Geometry: final body of the model. Coordinates: model frame, mm. Face numbers are marked on the shaded views. A direction names the side the tool comes from. Coordinates: 2 decimals unless noted, no trailing zeros. Loops run counter-clockwise (first coordinate to the right, second up) from the corner with the lowest first, then second, coordinate; pieces in that order, holes last. Notation, with made-up numbers: (-23.75, -11) -> (7.25, -11) arc R20 ccw to (7.25, 23) -> close; hole circle Ø10 at (70, 42.25). An arc over 180 degrees is marked (long way). One line per item, written item: value. Start each with the question number.
Item 1: Contact query for flat-ended pins moving along their axis: pin 1 Ø3 at (x, y) = (29, -34) entering from +Z; pin 2 Ø3 at (x, z) = (-4, 28) entering from -Y; pin 3 Ø2 at (x, y) = (47.5, -15) entering from -Z; pin 4 Ø15 at (x, z) = (0, 0) entering from -Y. Output: stop coordinate, or through.
Item 2: Section query D-D on z = -17. Return loops of the section in (x, y).
Item 3: Section query A-A on x = 0. Return loops of the section in (y, z), then the cut area to 3 significant figures.
Item 4: Mould query, pull axis Y, two halves, no side actions, for the marked faces 5, 6, 7 and 8. Classes: +Y half, -Y half, draft (parallel to the pull), parting line (faces both ways), or undercut.
Item 5: Section query C-C on y = -25.4. Give the number of separate pieces and of enclosed holes in the cut face, then the cut area to 3 significant figures.
Item 6: Set-up query: the marked faces 1, 2, 3 and 4. Return all of +Z, -Z, +X, -X, +Y, -Y with unobstructed straight access to the full face (end or side cutting, diameter ignored); none if empty.
Item 7: Ray query, probe 1 along Y at (x, z) = (0, 96); probe 2 along Z at (x, y) = (88, -27); probe 3 along X at (y, z) = (-25, 76). Return the intervals inside material, ascending. Write a range as from..to.
Item 8: Section query B-B on z = 68. Return loops of the section in (x, y).
from build123d import *

# Parameters (mm, degrees)
F1_DEPTH  = 50.8
F2_R      = 63.5
F3_DEPTH  = 49.53
F4_R      = 8.3185
F5_DEPTH  = 25.4
F9_R      = 19.05
F11_DEPTH = 76.2
F10_R     = 19.05
F12_DEPTH = 76.2
F6_R      = 19.05
F13_DEPTH = 76.2
F7_R      = 19.05
F14_DEPTH = 76.2
F8_R      = 19.05
F15_DEPTH = 76.2
F16_R     = 19.05


# Not quite as in the source:
# - a feature names something its author has since deleted; it is built from what else it names


with BuildPart() as f1:
    # F0 (on Front) → F1 (new body)
    with BuildSketch(Plane.XZ):
        Polygon((-23.0722505283, 63.5), (-46.1354505283, 63.5), (-53.262371273, 41.5655933534), (-113.6544600578, 61.1881724962), (-127.9083015471, 17.319359203), (-67.5218062965, -2.3204350678), (-74.6487270411, -24.2548417144), (-55.9902062965, -37.8110505451), (-93.314569817, -89.1836296879), (-55.9828842652, -116.3066868834), (-18.6585207447, -64.9341077406), (0, -78.4903165712), (18.6585207447, -64.9341077406), (55.9828842652, -116.3066868834), (93.2999257546, -89.194269222), (55.9902062965, -37.8110505451), (74.6487270411, -24.2548417144), (67.5218062965, -2.3204350678), (127.9138950812, 17.302144075), (113.6564223157, 61.1821332873), (53.2643335309, 41.5595541445), (46.1354505283, 63.5), (23.0722505283, 63.5), (23.0722505283, 127), (-23.0722505283, 127), align=None)
    extrude(amount=F1_DEPTH)

    # F2 (on face) → F3 (cut)
    with BuildSketch(Plane.XZ.offset(50.8)):
        Circle(F2_R)
    extrude(amount=-F3_DEPTH, mode=Mode.SUBTRACT)

    # F4 (on face) → F5 (cut)
    with BuildSketch(Plane(origin=(0, 0, 0), x_dir=(-1, 0, 0), z_dir=(0, 1, 0))):
        Circle(F4_R)
    extrude(amount=-F5_DEPTH, mode=Mode.SUBTRACT)

    # F9 (on face) → F11 (cut)
    with BuildSketch(Plane(origin=(-74.6487270411, 0, -102.7451582856), x_dir=(0.8090169944, 0, -0.5877852523), z_dir=(-0.5877852523, 0, -0.8090169944))):
        with Locations((0, 25.4)):
            Circle(F9_R)
    extrude(amount=-F11_DEPTH, mode=Mode.SUBTRACT)

    # F10 (on face) → F12 (cut)
    with BuildSketch(Plane(origin=(-120.7841775695, 0, 39.2451582856), x_dir=(0, -1, 0), z_dir=(-0.9510565163, 0, 0.3090169944))):
        with Locations((25.4, 0)):
            Circle(F10_R)
    extrude(amount=-F12_DEPTH, mode=Mode.SUBTRACT)

    # F6 (on face) → F13 (cut)
    with BuildSketch(Plane.XY.offset(127)):
        with Locations((0, -25.4)):
            Circle(F6_R)
    extrude(amount=-F13_DEPTH, mode=Mode.SUBTRACT)

    # F7 (on face) → F14 (cut)
    with BuildSketch(Plane(origin=(120.7841775695, 0, 39.2451582856), x_dir=(0, 1, 0), z_dir=(0.9510565163, 0, 0.3090169944))):
        with Locations((-25.4, 0)):
            Circle(F7_R)
    extrude(amount=-F14_DEPTH, mode=Mode.SUBTRACT)

    # F8 (on face) → F15 (cut)
    with BuildSketch(Plane(origin=(74.6487270411, 0, -102.7451582856), x_dir=(0.8090169944, 0, 0.5877852523), z_dir=(0.5877852523, 0, -0.8090169944))):
        with Locations((0, 25.4)):
            Circle(F8_R)
    extrude(amount=-F15_DEPTH, mode=Mode.SUBTRACT)

    # F16
    f16_edges = [f1.edges().sort_by_distance(p)[0] for p in [
        (0, -25.4, -78.490317),
        (74.648727, -25.4, -24.254842),
        (-74.648727, -25.4, -24.254842),
        (-46.135451, -25.4, 63.5),
        (46.135451, -25.4, 63.5),
    ]]
    fillet(f16_edges, radius=F16_R)


solid = f1.part
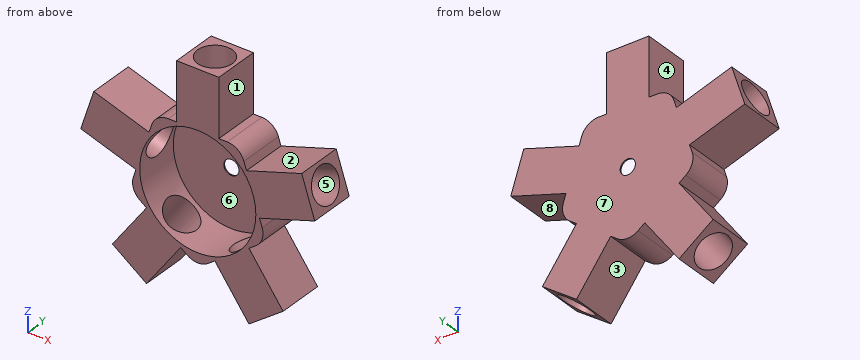
Reply:
1. pin 1: stops at z = 63.5
1. pin 2: stops at y = -1.27
1. pin 3: stops at z = -106.01
1. pin 4: passes through
2. outline: (-71.3, -50.8) -> (-61.18, -50.8) -> (-61.18, -1.27) -> (61.18, -1.27) -> (61.18, -50.8) -> (71.3, -50.8) -> (71.3, 0) -> (-71.3, 0) -> close
3. outline: (-50.8, -73.99) -> (0, -73.99) -> (0, -8.32) -> (-1.27, -8.32) -> (-1.27, -63.5) -> (-50.8, -63.5) -> close; (-50.8, 63.5) -> (-44.45, 63.5) -> (-44.45, 127) -> (-50.8, 127) -> close; (-6.35, 63.5) -> (-1.27, 63.5) -> (-1.27, 8.32) -> (0, 8.32) -> (0, 127) -> (-6.35, 127) -> close
3. area: 1,480 mm²
4. face 5: undercut
4. face 6: -Y half
4. face 7: +Y half
4. face 8: draft
5. separate pieces: 5
5. enclosed holes: 0
5. area: 4,170 mm²
6. face 1: +Z, +X, +Y, -Y
6. face 2: +Z, +Y, -Y
6. face 3: -Z, +Y, -Y
6. face 4: +Z, -X, +Y, -Y
7. probe 1: y = -50.8..-44.45, -6.35..0
7. probe 2: z = -88.83..-81.9, 4.33..8.63, 48.55..52.85
7. probe 3: x = -23.07..-19.05, 19.05..23.07
8. outline: (-23.07, -50.8) -> (23.07, -50.8) -> (23.07, 0) -> (-23.07, 0) -> close; hole circle Ø38.1 at (0, -25.4)
